Model file for the job. Use its own axes, mm. Coordinates: 2 decimals unless noted, no trailing zeros. Write each loop counter-clockwise with the first axis right and the second up, starting at its lowest first coordinate (ties: lowest second). Pieces come first, ordered by that corner, then holes. Notation, with made-up numbers: M -32,28.5 L -24,28.5 A17 ccw -24,54.5 Z; hole C 70,-7 d9. An arc over 180 degrees is marked long. Use CSV: the item, a comma, the result in double quotes. Start each with the question number.
from build123d import *

# Parameters (mm, degrees)
F0_W          = 94.60038
F0_H          = 92.940778
F1_DEPTH      = 101.6
F1_DEPTH_BACK = 50.8
F2_R          = 25.4
F3_SIZE       = 2.54
F4_R          = 27.414742
F5_DEPTH      = 138.78718
F6_SIZE       = 5.08


with BuildPart() as f1:
    # F0 (on Top) → F1 (new body, two sides)
    with BuildSketch(Plane.XY) as f1_sk:
        Rectangle(F0_W, F0_H)
    extrude(amount=F1_DEPTH)
    extrude(f1_sk.sketch, amount=-F1_DEPTH_BACK)

    # F2
    f2_edges = [f1.edges().sort_by_distance(p)[0] for p in [
        (-47.30019, 0, 101.6),
        (47.30019, 0, 101.6),
        (-47.30019, 0, -50.8),
        (47.30019, 0, -50.8),
    ]]
    fillet(f2_edges, radius=F2_R)

    # F3
    f3_edges = [f1.edges().sort_by_distance(p)[0] for p in [
        (47.30019, 46.470389, 25.4),
        (47.30019, -46.470389, 25.4),
    ]]
    chamfer(f3_edges, length=F3_SIZE)

    # F4 (on face) → F5 (cut)
    with BuildSketch(Plane(origin=(0, 46.470389, 0), x_dir=(-1, 0, 0), z_dir=(0, 1, 0))):
        Circle(F4_R)
    extrude(amount=-F5_DEPTH, mode=Mode.SUBTRACT)

    # F6
    f6_edges = [f1.edges().sort_by_distance(p)[0] for p in [
        (27.414742, -46.470389, 0),
        (27.414742, 46.470389, 0),
    ]]
    chamfer(f6_edges, length=F6_SIZE)


solid = f1.part
1) Two-plate mould, pull along X, no slides. Class faces 1 (the face through (-37.997, -46.311, 92.655)), 2 (the face through (21.951, 41.637, -16.832)), 3 (the face through (-14.738, 0.579, 23.116)), 4 (the face through (47.3, -1, 26)): pulls with the +X half, pulls with the -X half, needs draft (parallel to the pull), parting line crosses it, or undercut.
2) Band-saw the part on C-C on x = 0. List the corners of the cut face in (y, z), then the cut area to 3 significant figures.
3) Wall check: L1, parallel to Z at x = 0, y = -22; L2, parallel to X at y = 16, z = 8.5; L3, parallel to X at y = -10, z = 2.5. Give the ranges that are in metal, low to high. Write a range as [from, to].
4) Band-saw the part on B-B on y = -19. List the corners of the cut face in (x, z).
5) Band-saw the part on A-A on z = 0. List the corners of the cut face in (x, y).
6) Drop a flat-ended pin along its axis: P1, Ø8, axis at y = -29, z = -32, coming from the +X side. Give the stop position or say it passes through.
Findings below:
1,face 1,"pulls with the -X half"
1,face 2,"undercut"
1,face 3,"undercut"
1,face 4,"pulls with the +X half"
2,outline,"M -46.47,-48.26 L -43.93,-50.8 L 43.93,-50.8 L 46.47,-48.26 L 46.47,-32.49 L 41.39,-27.41 L -41.39,-27.41 L -46.47,-32.49 Z; M -46.47,32.49 L -41.39,27.41 L 41.39,27.41 L 46.47,32.49 L 46.47,99.06 L 43.93,101.6 L -43.93,101.6 L -46.47,99.06 Z"
2,area,"9,000 mm2"
3,L1,"z = [-50.8, -27.41], [27.41, 101.6]"
3,L2,"x = [-47.3, -26.06], [26.06, 47.3]"
3,L3,"x = [-47.3, -27.3], [27.3, 47.3]"
4,outline,"M -47.3,-25.4 A25.4 ccw -21.9,-50.8 L 21.9,-50.8 A25.4 ccw 47.3,-25.4 L 47.3,76.2 A25.4 ccw 21.9,101.6 L -21.9,101.6 A25.4 ccw -47.3,76.2 Z; hole C 0,0 d54.83"
5,outline,"M -47.3,-43.93 L -44.76,-46.47 L -32.49,-46.47 L -27.41,-41.39 L -27.41,41.39 L -32.49,46.47 L -44.76,46.47 L -47.3,43.93 Z; M 27.41,-41.39 L 32.49,-46.47 L 44.76,-46.47 L 47.3,-43.93 L 47.3,43.93 L 44.76,46.47 L 32.49,46.47 L 27.41,41.39 Z"
6,P1,"stops at x = 47.17"
